Model file for the job. Use its own axes, mm. Coordinates: 2 decimals unless noted, no trailing zeros. Return JSON: item names as keys, results as strings. Group by question number.
1) Pull direction Y, two halves, no side cores. Call faces 1 (the flat face through (39, 41, 0)), 2 (the cylindrical face through (68.504, 10.195, 0.198)): +Y half, -Y half, draft (parallel to the pull), parting line (faces both ways), or undercut.
2) Probe line 1 (X direction, y = 42.5, z = 0.15) (3 decimals); line 2 (X direction, y = 22, z = 0.1) (3 decimals). List the from-to ranges inside material, lowest first.
3) Flat gauge pin, fed straight in: pin 1 (0.7 mm diameter, centred on x = 28.57, y = 57.78, fed in from -Z). Where does the tip first touch, or does it go through?
from build123d import *

# Parameters (mm, degrees)
BOARD_DEPTH                 = 0.39116
ESBO_O2_R                   = 0.6
HOLE_P1_1_DEPTH             = 0.39116
ESBO_O3_R                   = 0.6
HOLE_P1_2_DEPTH             = 1.39116
ESBO_O4_R                   = 0.6
HOLE_P3_12_DEPTH            = 1.39116
ESBO_O5_R                   = 0.6
HOLE_P3_13_DEPTH            = 1.39116
ESBO_O6_R                   = 0.6
HOLE_P3_14_DEPTH            = 1.39116
ESBO_O7_R                   = 0.6
HOLE_P3_15_DEPTH            = 1.39116
ESBO_O8_R                   = 0.6
HOLE_P3_11_DEPTH            = 1.39116
ESBO_O9_R                   = 0.6
HOLE_P3_10_DEPTH            = 1.39116
ESBO_O10_R                  = 0.6
HOLE_P3_9_DEPTH             = 1.39116
ESBO_O11_R                  = 0.6
HOLE_P3_8_DEPTH             = 1.39116
ESBO_O12_R                  = 0.6
HOLE_P3_7_DEPTH             = 1.39116
ESBO_O13_R                  = 0.6
HOLE_P3_6_DEPTH             = 1.39116
ESBO_O14_R                  = 0.6
HOLE_P3_5_DEPTH             = 1.39116
ESBO_O15_R                  = 0.6
HOLE_P3_1_DEPTH             = 1.39116
ESBO_O16_R                  = 0.6
HOLE_P3_2_DEPTH             = 1.39116
ESBO_O17_R                  = 0.6
HOLE_P3_3_DEPTH             = 1.39116
ESBO_O18_R                  = 0.6
HOLE_P3_4_DEPTH             = 1.39116
ESBO_O19_R                  = 0.6
HOLE_P2_12_DEPTH            = 1.39116
ESBO_O20_R                  = 0.6
HOLE_P2_13_DEPTH            = 1.39116
ESBO_O21_R                  = 0.6
HOLE_P2_14_DEPTH            = 1.39116
ESBO_O22_R                  = 0.6
HOLE_P2_15_DEPTH            = 1.39116
ESBO_O23_R                  = 0.6
HOLE_P2_11_DEPTH            = 1.39116
ESBO_O24_R                  = 0.6
HOLE_P2_10_DEPTH            = 1.39116
ESBO_O25_R                  = 0.6
HOLE_P2_9_DEPTH             = 1.39116
ESBO_O26_R                  = 0.6
HOLE_P2_8_DEPTH             = 1.39116
ESBO_O27_R                  = 0.6
HOLE_P2_7_DEPTH             = 1.39116
ESBO_O28_R                  = 0.6
HOLE_P2_6_DEPTH             = 1.39116
ESBO_O29_R                  = 0.6
HOLE_P2_5_DEPTH             = 1.39116
ESBO_O30_R                  = 0.6
HOLE_P2_1_DEPTH             = 1.39116
ESBO_O31_R                  = 0.6
HOLE_P2_2_DEPTH             = 1.39116
ESBO_O32_R                  = 0.6
HOLE_P2_3_DEPTH             = 1.39116
ESBO_O33_R                  = 0.6
HOLE_P2_4_DEPTH             = 1.39116
ESBO_O34_R                  = 1.5
FREE_CORTE_EXTRUS_O33_DEPTH = 10


with BuildPart() as part:
    # Esboço1 → Board (new body)
    with BuildSketch(Plane.XY):
        Polygon((0, 0), (80.00499, 0), (80.00499, 80.25899), (0, 80.259), align=None)
    extrude(amount=BOARD_DEPTH)

    # Esboço2 → Hole - P1-1 (cut)
    with BuildSketch(Plane.XY.offset(0.39116)):
        with Locations((60, 37.5)):
            Circle(ESBO_O2_R)
    extrude(amount=-HOLE_P1_1_DEPTH, mode=Mode.SUBTRACT)

    # Esboço3 → Hole - P1-2 (cut, through all)
    with BuildSketch(Plane.XY.offset(0.39116)):
        with Locations((60, 42.5)):
            Circle(ESBO_O3_R)
    extrude(amount=-HOLE_P1_2_DEPTH, mode=Mode.SUBTRACT)

    # Esboço4 → Hole - P3-12 (cut, through all)
    with BuildSketch(Plane.XY.offset(0.39116)):
        with Locations((51.43, 50.16)):
            Circle(ESBO_O4_R)
    extrude(amount=-HOLE_P3_12_DEPTH, mode=Mode.SUBTRACT)

    # Esboço5 → Hole - P3-13 (cut, through all)
    with BuildSketch(Plane.XY.offset(0.39116)):
        with Locations((51.43, 52.7)):
            Circle(ESBO_O5_R)
    extrude(amount=-HOLE_P3_13_DEPTH, mode=Mode.SUBTRACT)

    # Esboço6 → Hole - P3-14 (cut, through all)
    with BuildSketch(Plane.XY.offset(0.39116)):
        with Locations((51.43, 55.24)):
            Circle(ESBO_O6_R)
    extrude(amount=-HOLE_P3_14_DEPTH, mode=Mode.SUBTRACT)

    # Esboço7 → Hole - P3-15 (cut, through all)
    with BuildSketch(Plane.XY.offset(0.39116)):
        with Locations((51.43, 57.78)):
            Circle(ESBO_O7_R)
    extrude(amount=-HOLE_P3_15_DEPTH, mode=Mode.SUBTRACT)

    # Esboço8 → Hole - P3-11 (cut, through all)
    with BuildSketch(Plane.XY.offset(0.39116)):
        with Locations((51.43, 47.62)):
            Circle(ESBO_O8_R)
    extrude(amount=-HOLE_P3_11_DEPTH, mode=Mode.SUBTRACT)

    # Esboço9 → Hole - P3-10 (cut, through all)
    with BuildSketch(Plane.XY.offset(0.39116)):
        with Locations((51.43, 45.08)):
            Circle(ESBO_O9_R)
    extrude(amount=-HOLE_P3_10_DEPTH, mode=Mode.SUBTRACT)

    # Esboço10 → Hole - P3-9 (cut, through all)
    with BuildSketch(Plane.XY.offset(0.39116)):
        with Locations((51.43, 42.54)):
            Circle(ESBO_O10_R)
    extrude(amount=-HOLE_P3_9_DEPTH, mode=Mode.SUBTRACT)

    # Esboço11 → Hole - P3-8 (cut, through all)
    with BuildSketch(Plane.XY.offset(0.39116)):
        with Locations((51.43, 40)):
            Circle(ESBO_O11_R)
    extrude(amount=-HOLE_P3_8_DEPTH, mode=Mode.SUBTRACT)

    # Esboço12 → Hole - P3-7 (cut, through all)
    with BuildSketch(Plane.XY.offset(0.39116)):
        with Locations((51.43, 37.46)):
            Circle(ESBO_O12_R)
    extrude(amount=-HOLE_P3_7_DEPTH, mode=Mode.SUBTRACT)

    # Esboço13 → Hole - P3-6 (cut, through all)
    with BuildSketch(Plane.XY.offset(0.39116)):
        with Locations((51.43, 34.92)):
            Circle(ESBO_O13_R)
    extrude(amount=-HOLE_P3_6_DEPTH, mode=Mode.SUBTRACT)

    # Esboço14 → Hole - P3-5 (cut, through all)
    with BuildSketch(Plane.XY.offset(0.39116)):
        with Locations((51.43, 32.38)):
            Circle(ESBO_O14_R)
    extrude(amount=-HOLE_P3_5_DEPTH, mode=Mode.SUBTRACT)

    # Esboço15 → Hole - P3-1 (cut, through all)
    with BuildSketch(Plane.XY.offset(0.39116)):
        with Locations((51.43, 22.22)):
            Circle(ESBO_O15_R)
    extrude(amount=-HOLE_P3_1_DEPTH, mode=Mode.SUBTRACT)

    # Esboço16 → Hole - P3-2 (cut, through all)
    with BuildSketch(Plane.XY.offset(0.39116)):
        with Locations((51.43, 24.76)):
            Circle(ESBO_O16_R)
    extrude(amount=-HOLE_P3_2_DEPTH, mode=Mode.SUBTRACT)

    # Esboço17 → Hole - P3-3 (cut, through all)
    with BuildSketch(Plane.XY.offset(0.39116)):
        with Locations((51.43, 27.3)):
            Circle(ESBO_O17_R)
    extrude(amount=-HOLE_P3_3_DEPTH, mode=Mode.SUBTRACT)

    # Esboço18 → Hole - P3-4 (cut, through all)
    with BuildSketch(Plane.XY.offset(0.39116)):
        with Locations((51.43, 29.84)):
            Circle(ESBO_O18_R)
    extrude(amount=-HOLE_P3_4_DEPTH, mode=Mode.SUBTRACT)

    # Esboço19 → Hole - P2-12 (cut, through all)
    with BuildSketch(Plane.XY.offset(0.39116)):
        with Locations((28.57, 50.16)):
            Circle(ESBO_O19_R)
    extrude(amount=-HOLE_P2_12_DEPTH, mode=Mode.SUBTRACT)

    # Esboço20 → Hole - P2-13 (cut, through all)
    with BuildSketch(Plane.XY.offset(0.39116)):
        with Locations((28.57, 52.7)):
            Circle(ESBO_O20_R)
    extrude(amount=-HOLE_P2_13_DEPTH, mode=Mode.SUBTRACT)

    # Esboço21 → Hole - P2-14 (cut, through all)
    with BuildSketch(Plane.XY.offset(0.39116)):
        with Locations((28.57, 55.24)):
            Circle(ESBO_O21_R)
    extrude(amount=-HOLE_P2_14_DEPTH, mode=Mode.SUBTRACT)

    # Esboço22 → Hole - P2-15 (cut, through all)
    with BuildSketch(Plane.XY.offset(0.39116)):
        with Locations((28.57, 57.78)):
            Circle(ESBO_O22_R)
    extrude(amount=-HOLE_P2_15_DEPTH, mode=Mode.SUBTRACT)

    # Esboço23 → Hole - P2-11 (cut, through all)
    with BuildSketch(Plane.XY.offset(0.39116)):
        with Locations((28.57, 47.62)):
            Circle(ESBO_O23_R)
    extrude(amount=-HOLE_P2_11_DEPTH, mode=Mode.SUBTRACT)

    # Esboço24 → Hole - P2-10 (cut, through all)
    with BuildSketch(Plane.XY.offset(0.39116)):
        with Locations((28.57, 45.08)):
            Circle(ESBO_O24_R)
    extrude(amount=-HOLE_P2_10_DEPTH, mode=Mode.SUBTRACT)

    # Esboço25 → Hole - P2-9 (cut, through all)
    with BuildSketch(Plane.XY.offset(0.39116)):
        with Locations((28.57, 42.54)):
            Circle(ESBO_O25_R)
    extrude(amount=-HOLE_P2_9_DEPTH, mode=Mode.SUBTRACT)

    # Esboço26 → Hole - P2-8 (cut, through all)
    with BuildSketch(Plane.XY.offset(0.39116)):
        with Locations((28.57, 40)):
            Circle(ESBO_O26_R)
    extrude(amount=-HOLE_P2_8_DEPTH, mode=Mode.SUBTRACT)

    # Esboço27 → Hole - P2-7 (cut, through all)
    with BuildSketch(Plane.XY.offset(0.39116)):
        with Locations((28.57, 37.46)):
            Circle(ESBO_O27_R)
    extrude(amount=-HOLE_P2_7_DEPTH, mode=Mode.SUBTRACT)

    # Esboço28 → Hole - P2-6 (cut, through all)
    with BuildSketch(Plane.XY.offset(0.39116)):
        with Locations((28.57, 34.92)):
            Circle(ESBO_O28_R)
    extrude(amount=-HOLE_P2_6_DEPTH, mode=Mode.SUBTRACT)

    # Esboço29 → Hole - P2-5 (cut, through all)
    with BuildSketch(Plane.XY.offset(0.39116)):
        with Locations((28.57, 32.38)):
            Circle(ESBO_O29_R)
    extrude(amount=-HOLE_P2_5_DEPTH, mode=Mode.SUBTRACT)

    # Esboço30 → Hole - P2-1 (cut, through all)
    with BuildSketch(Plane.XY.offset(0.39116)):
        with Locations((28.57, 22.22)):
            Circle(ESBO_O30_R)
    extrude(amount=-HOLE_P2_1_DEPTH, mode=Mode.SUBTRACT)

    # Esboço31 → Hole - P2-2 (cut, through all)
    with BuildSketch(Plane.XY.offset(0.39116)):
        with Locations((28.57, 24.76)):
            Circle(ESBO_O31_R)
    extrude(amount=-HOLE_P2_2_DEPTH, mode=Mode.SUBTRACT)

    # Esboço32 → Hole - P2-3 (cut, through all)
    with BuildSketch(Plane.XY.offset(0.39116)):
        with Locations((28.57, 27.3)):
            Circle(ESBO_O32_R)
    extrude(amount=-HOLE_P2_3_DEPTH, mode=Mode.SUBTRACT)

    # Esboço33 → Hole - P2-4 (cut, through all)
    with BuildSketch(Plane.XY.offset(0.39116)):
        with Locations((28.57, 29.84)):
            Circle(ESBO_O33_R)
    extrude(amount=-HOLE_P2_4_DEPTH, mode=Mode.SUBTRACT)

    # Esboço34 → Free-Corte-extrusão33 (cut)
    with BuildSketch(Plane.XY.offset(0.39116)):
        with Locations((10.002495, 70.129495)):
            Circle(ESBO_O34_R)
        with Locations((70.002495, 70.129495)):
            Circle(ESBO_O34_R)
        with Locations((70.002495, 10.129495)):
            Circle(ESBO_O34_R)
        with Locations((10.002495, 10.129495)):
            Circle(ESBO_O34_R)
    extrude(amount=-FREE_CORTE_EXTRUS_O33_DEPTH, mode=Mode.SUBTRACT)


solid = part.part
Answers below:
{
 "1": {"face 1": "draft", "face 2": "undercut"},
 "2": {"line 1": "x = 0 to 27.971, 29.169 to 50.831, 52.029 to 59.4, 60.6 to 80.005", "line 2": "x = 0 to 28.012, 29.128 to 50.872, 51.988 to 80.005"},
 "3": {"pin 1": "passes through"}
}
